from build123d import *

# Parameters (mm, degrees)
ESQUISSE1_W                  = 203.2
ESQUISSE1_H                  = 203.2
BOSS_EXTRU_1_DEPTH           = 6.35
ESQUISSE2_R                  = 4
ENL_V_MAT_EXTRU_1_DEPTH      = 144.824345992
ENL_V_MAT_EXTRU_2_DEPTH      = 144.824345992
ENL_V_MAT_EXTRU_3_DEPTH      = 144.824345992
CONG_1_R                     = 5
ESQUISSE5_R                  = 2.5
ENL_V_MAT_EXTRU_4_DEPTH      = 144.824345992
ESQUISSE6_R                  = 2.5
ENL_V_MAT_EXTRU_5_DEPTH      = 144.824345992
ENL_V_MAT_EXTRU_6_DEPTH      = 144.824345992
ENL_V_MAT_EXTRU_6_DEPTH_BACK = 144.824345992
ESQUISSE8_R                  = 2.5
ENL_V_MAT_EXTRU_7_DEPTH      = 144.824345992


with BuildPart() as part:
    # Esquisse1 → Boss.-Extru.1 (new body)
    with BuildSketch(Plane(origin=(0, 0, 0), x_dir=(1, 0, 0), z_dir=(0, 1, 0))):
        Rectangle(ESQUISSE1_W, ESQUISSE1_H)
    extrude(amount=BOSS_EXTRU_1_DEPTH)

    # Esquisse2 → Enl_v. mat.-Extru.1 (cut, through all)
    with BuildSketch(Plane(origin=(0, 6.35, 0), x_dir=(1, 0, 0), z_dir=(0, 1, 0))):
        with Locations(Location((-75, 65, 0), (0, 0, 270))):
            Circle(ESQUISSE2_R)
        with Locations(Location((75, 65, 0), (0, 0, 270))):
            Circle(ESQUISSE2_R)
        with Locations(Location((0, -65, 0), (0, 0, 270))):
            Circle(ESQUISSE2_R)
    extrude(amount=-ENL_V_MAT_EXTRU_1_DEPTH, mode=Mode.SUBTRACT)

    # Esquisse3 → Enl_v. mat.-Extru.2 (cut, through all)
    with BuildSketch(Plane(origin=(0, 6.35, 0), x_dir=(1, 0, 0), z_dir=(0, 1, 0))):
        Polygon((-17.05, 86.15), (-21.15, 82.05), (-21.15, 47.95), (-17.05, 43.85), (17.05, 43.85), (21.15, 47.95), (21.15, 82.05), (17.05, 86.15), align=None)
    extrude(amount=-ENL_V_MAT_EXTRU_2_DEPTH, mode=Mode.SUBTRACT)

    # Esquisse4 → Enl_v. mat.-Extru.3 (cut, through all)
    with BuildSketch(Plane(origin=(0, 6.35, 0), x_dir=(1, 0, 0), z_dir=(0, 1, 0))):
        Polygon((-49.6, -101.6), (-39.6, -101.6), (-39.6, 59), (-21.15, 59), (-21.15, 71), (-49.6, 71), align=None)
    extrude(amount=-ENL_V_MAT_EXTRU_3_DEPTH, mode=Mode.SUBTRACT)

    # Cong_1
    cong_1_edges = [part.edges().sort_by_distance(p)[0] for p in [
        (-49.6, 3.175, -71),
        (-39.6, 3.175, -59),
    ]]
    fillet(cong_1_edges, radius=CONG_1_R)

    # Esquisse5 → Enl_v. mat.-Extru.4 (cut, through all)
    with BuildSketch(Plane(origin=(0, 6.35, 0), x_dir=(1, 0, 0), z_dir=(0, 1, 0))):
        with Locations(Location((-33.425, 49.85, 0), (0, 0, 270))):
            Circle(ESQUISSE5_R)
        with Locations(Location((-33.425, 79.85, 0), (0, 0, 270))):
            Circle(ESQUISSE5_R)
        with Locations(Location((33.725, 79.85, 0), (0, 0, 270))):
            Circle(ESQUISSE5_R)
        with Locations(Location((33.725, 49.85, 0), (0, 0, 270))):
            Circle(ESQUISSE5_R)
    extrude(amount=-ENL_V_MAT_EXTRU_4_DEPTH, mode=Mode.SUBTRACT)

    # Esquisse6 → Enl_v. mat.-Extru.5 (cut, through all)
    with BuildSketch(Plane(origin=(0, 6.35, 0), x_dir=(1, 0, 0), z_dir=(0, 1, 0))):
        with Locations(Location((93.6, -93.6, 0), (0, 0, 270))):
            Circle(ESQUISSE6_R)
        with Locations(Location((-93.6, -93.6, 0), (0, 0, 270))):
            Circle(ESQUISSE6_R)
        with Locations(Location((-93.6, 93.6, 0), (0, 0, 270))):
            Circle(ESQUISSE6_R)
        with Locations(Location((93.6, 93.6, 0), (0, 0, 270))):
            Circle(ESQUISSE6_R)
    extrude(amount=-ENL_V_MAT_EXTRU_5_DEPTH, mode=Mode.SUBTRACT)

    # Esquisse7 → Enl_v. mat.-Extru.6 (cut, two sides: drawn at the far end of the back side and taken through both)
    with BuildSketch(Plane(origin=(0, 6.35, 0), x_dir=(1, 0, 0), z_dir=(0, 1, 0)).offset(-ENL_V_MAT_EXTRU_6_DEPTH_BACK)):
        Polygon((-98.172614132, -93.6), (-95.886307066, -97.56), (-91.313692934, -97.56), (-89.027385868, -93.6), (-91.313692934, -89.64), (-95.886307066, -89.64), align=None)
        Polygon((89.027385868, -93.6), (91.313692934, -97.56), (95.886307066, -97.56), (98.172614132, -93.6), (95.886307066, -89.64), (91.313692934, -89.64), align=None)
        Polygon((89.027385868, 93.6), (91.313692934, 89.64), (95.886307066, 89.64), (98.172614132, 93.6), (95.886307066, 97.56), (91.313692934, 97.56), align=None)
        Polygon((-98.172614132, 93.6), (-95.886307066, 89.64), (-91.313692934, 89.64), (-89.027385868, 93.6), (-91.313692934, 97.56), (-95.886307066, 97.56), align=None)
    extrude(amount=ENL_V_MAT_EXTRU_6_DEPTH + ENL_V_MAT_EXTRU_6_DEPTH_BACK, mode=Mode.SUBTRACT)

    # Esquisse8 → Enl_v. mat.-Extru.7 (cut, through all)
    with BuildSketch(Plane(origin=(0, 6.35, 0), x_dir=(1, 0, 0), z_dir=(0, 1, 0))):
        with Locations(Location((90.588457268, 56, 0), (0, 0, 270))):
            Circle(ESQUISSE8_R)
        with Locations(Location((59.411542732, 56, 0), (0, 0, 270))):
            Circle(ESQUISSE8_R)
        with Locations(Location((75, 83, 0), (0, 0, 270))):
            Circle(ESQUISSE8_R)
        with Locations(Location((-90.588457268, 56, 0), (0, 0, 270))):
            Circle(ESQUISSE8_R)
        with Locations(Location((-75, 83, 0), (0, 0, 270))):
            Circle(ESQUISSE8_R)
        with Locations(Location((-59.411542732, 56, 0), (0, 0, 270))):
            Circle(ESQUISSE8_R)
        with Locations(Location((15.588457268, -74, 0), (0, 0, 270))):
            Circle(ESQUISSE8_R)
        with Locations(Location((-15.588457268, -74, 0), (0, 0, 270))):
            Circle(ESQUISSE8_R)
        with Locations(Location((0, -47, 0), (0, 0, 270))):
            Circle(ESQUISSE8_R)
    extrude(amount=-ENL_V_MAT_EXTRU_7_DEPTH, mode=Mode.SUBTRACT)


solid = part.part
Geometry: final body of the model. Coordinates: model frame, mm. A direction names the side the tool comes from. Round coordinates to 2 decimals unless told otherwise and drop trailing zeros. Loops run counter-clockwise (first coordinate to the right, second up) from the corner with the lowest first, then second, coordinate; pieces in that order, holes last. Notation, with made-up numbers: M -36,7 L -18,7 A18 cw -18,34 Z; hole C 64.25,40 d4. An arc over 180 degrees is marked long. Put each result on its own line as item: value. Start each with the question number.
(1) Set-up query: faces 1 (the face through (-21.15, 3, -77)), 2 (the face through (30, 3, 101.6)). Return all of +Z, -Z, +X, -X, +Y, -Y with unobstructed straight access to the full face (end or side cutting, diameter ignored); none if empty.
(2) Section query C-C (z = 47). Return loops of the section in (x, y).
(3) Material intervals for line 1 along X through (y, z) = (3.75, 47); line 2 along X through (y, z) = (3.75, -65); line 3 along X through (y, z) = (3.25, 65), sorted ascending. Write a range as [from, to].
(4) Section query D-D (x = -8). Return loops of the section in (y, z).
(5) Draft query along Z for faces 3 (the face through (-101.6, 3, 1)), 4 (the face through (-76.5, 3.2, -85)), 5 (the face through (-48.17, 3.13, -69.5)). Return one class per face: +Z half, -Z half, draft (parallel to the pull), parting line (faces both ways), or undercut.
(6) Section query A-A (x = 75). Return loops of the section in (y, z).
(7) Section query B-B (z = 74). Return loops of the section in (x, y).
Findings below:
1. face 1: +Y, -Y
1. face 2: +Z, +X, -X, +Y, -Y
2. outline: M -101.6,0 L -49.6,0 L -49.6,6.35 L -101.6,6.35 Z; M -39.6,0 L -2.5,0 L -2.5,6.35 L -39.6,6.35 Z; M 2.5,0 L 101.6,0 L 101.6,6.35 L 2.5,6.35 Z
3. line 1: x = [-101.6, -49.6], [-39.6, -2.5], [2.5, 101.6]
3. line 2: x = [-101.6, -79], [-71, -49.6], [21.15, 71], [79, 101.6]
3. line 3: x = [-101.6, -49.6], [-39.6, -4], [4, 101.6]
4. outline: M 0,-101.6 L 6.35,-101.6 L 6.35,-86.15 L 0,-86.15 Z; M 0,-43.85 L 6.35,-43.85 L 6.35,101.6 L 0,101.6 Z
5. face 3: draft
5. face 4: undercut
5. face 5: +Z half
6. outline: M 0,-101.6 L 6.35,-101.6 L 6.35,-85.5 L 0,-85.5 Z; M 0,-80.5 L 6.35,-80.5 L 6.35,-69 L 0,-69 Z; M 0,-61 L 6.35,-61 L 6.35,101.6 L 0,101.6 Z
7. outline: M -101.6,0 L -49.6,0 L -49.6,6.35 L -101.6,6.35 Z; M -39.6,0 L -18.09,0 L -18.09,6.35 L -39.6,6.35 Z; M -13.09,0 L 13.09,0 L 13.09,6.35 L -13.09,6.35 Z; M 18.09,0 L 101.6,0 L 101.6,6.35 L 18.09,6.35 Z
